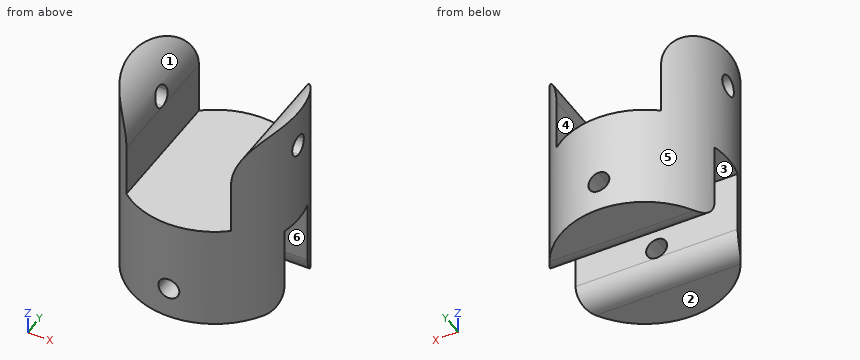
from build123d import *

# Parameters (mm, degrees)
F0_R        = 8
F1_DEPTH    = 10
F3_DEPTH    = 10
F5_DEPTH    = 8
F6_R        = 2
F7_T1_DEPTH = 37.4899959968
F9_DEPTH    = 12.5
F11_DEPTH   = 12.5


# Not quite as in the source:
# - a fillet or chamfer that OpenCascade refuses, or shapes differently, is made with other operations: its cross-section is extruded or revolved along the edge and cut away or added


with BuildPart() as f1:
    # F0 (on Top) → F1 (new body, symmetric)
    with BuildSketch(Plane.XY):
        Circle(F0_R)
    extrude(amount=F1_DEPTH, both=True)

    # F2 (on face) → F3 (cut)
    with BuildSketch(Plane.XY.offset(10)):
        with BuildLine():
            ThreePointArc((5, 6.2449979984), (0, 8), (-5, 6.2449979984))
            Line((-5, 6.2449979984), (-5, -6.2449979984))
            ThreePointArc((-5, -6.2449979984), (0, -8), (5, -6.2449979984))
            Line((5, -6.2449979984), (5, 6.2449979984))
        make_face()
    extrude(amount=-F3_DEPTH, mode=Mode.SUBTRACT)

    # F4 (on face) → F5 (cut)
    with BuildSketch(Plane(origin=(0, 0, -10), x_dir=(1, 0, 0), z_dir=(0, 0, -1))):
        with BuildLine():
            Line((7.7459666924, 2), (-7.7459666924, 2))
            ThreePointArc((-7.7459666924, 2), (-8, 0), (-7.7459666924, -2))
            Line((-7.7459666924, -2), (7.7459666924, -2))
            ThreePointArc((7.7459666924, -2), (7.9362375701, -1.0080343399), (8, 0))
            ThreePointArc((8, 0), (7.9362375701, 1.0080343399), (7.7459666924, 2))
        make_face()
    extrude(amount=-F5_DEPTH, mode=Mode.SUBTRACT)

    # F6
    f6_edges = [f1.edges().sort_by_distance(p)[0] for p in [
        (0, 2, -10),
        (0, -2, -10),
    ]]
    fillet(f6_edges, radius=F6_R)

    # F7: fillet of radius 5 on 2 edges, made by hand

    # F7_s2 → F7_t1 (cut)
    with BuildSketch(Plane.XZ.offset(-18.7449979984)):
        with BuildLine():
            ThreePointArc((-5, 5), (-6.4644660941, 8.5355339059), (-10, 10))
            Line((-10, 10), (-5, 10))
            Line((-5, 10), (-5, 5))
        make_face()
        with BuildLine():
            ThreePointArc((10, 10), (6.4644660941, 8.5355339059), (5, 5))
            Line((5, 5), (5, 10))
            Line((5, 10), (10, 10))
        make_face()
    extrude(amount=F7_T1_DEPTH, mode=Mode.SUBTRACT)

    # F8 (on Right) → F9 (cut, symmetric)
    with BuildSketch(Plane.YZ):
        with BuildLine():
            ThreePointArc((0, 5), (0.7071067812, 5.2928932188), (1, 6))
            ThreePointArc((1, 6), (-0.7071067812, 6.7071067812), (0, 5))
        make_face()
    extrude(amount=F9_DEPTH, both=True, mode=Mode.SUBTRACT)

    # F10 (on Front) → F11 (cut, symmetric)
    with BuildSketch(Plane.XZ):
        with BuildLine():
            ThreePointArc((0, -6), (-0.7071067812, -7.7071067812), (1, -7))
            ThreePointArc((1, -7), (0.7071067812, -6.2928932188), (0, -6))
        make_face()
    extrude(amount=F11_DEPTH, both=True, mode=Mode.SUBTRACT)


solid = f1.part
Check sheet for the modelled part. Datum: model origin and axes. Units: mm. Face numbers are marked on the shaded views. A direction names the side the tool comes from. Give positions to 0.01 mm unless a question says otherwise; leave off trailing zeros. Loops run counter-clockwise (first coordinate to the right, second up) from the corner with the lowest first, then second, coordinate; pieces in that order, holes last. Notation, with made-up numbers: M -17,-3 L 23,-3 A20 ccw 23,34 Z; hole C -13,-18.5 d11. An arc over 180 degrees is marked long. Answer as a JSON object with one key per item and string values. Group by question number.
Q1. Cross-section at C-C on x = -3.75. Record the cut outline in (y, z), then the cut area to 3 significant figures.
Q2. Cross-section at A-A on z = -2.25. Record the cut outline in (x, y), then the cut area to 3 significant figures.
Q3. Cross-section at B-B on y = 5.75. Record the cut outline in (x, z), then the cut area to 3 significant figures.
Q4. Cross-section at D-D on y = -1.5. Record the cut outline in (x, z), then the cut area to 3 significant figures.
Q5. Release check for a two-part mould opening along Y. For the marked faces 4, 5 and 6 record: released by +Y, released by -Y, zero draft, split by the parting line, or undercut.
Q6. Access from +Z, -Z, +X, -X, +Y, -Y to the whole of each face (thin tool, end or side, straight path). Record for the marked faces 1, 2 and 3.
Q7. Material ranges on line 1 along X through (y, z) = (-4, 3.25); line 2 along Z through (x, y) = (0, 6); line 3 along Z through (x, y) = (-6, 0), recorded low to high. Write a range as [from, to].
Q8. Go/stop test with flat-tipped pins: P1, Ø2.5, axis at y = 0, z = 6, coming from the -X side; P2, Ø2, axis at y = -4.5, z = 6, coming from the +X side; P3, Ø1, axis at x = -5, y = 2.5, coming from the -Z side; P4, Ø1, axis at x = -6, y = 3, coming from the +Z side. Record where each tip stops, or that it passes through.
Evaluation:
{
 "1": {"outline": "M -7.07,-10 L -4,-10 A2 ccw -2,-8 L -2,-2 L 2,-2 L 2,-8 A2 ccw 4,-10 L 7.07,-10 L 7.07,0 L -7.07,0 Z", "area": "108 mm2"},
 "2": {"outline": "M -7.75,-2 A8 ccw 7.75,-2 Z; M -7.75,2 L 7.75,2 A8 ccw Z", "area": "138 mm2"},
 "3": {"outline": "M -5.56,-10 L 5.56,-10 L 5.56,7.3 A5 ccw 5,5 L 5,0 L -5,0 L -5,5 A5 ccw -5.56,7.3 Z; hole C 0,-7 d2", "area": "115 mm2"},
 "4": {"outline": "M -7.86,-2 L 7.86,-2 L 7.86,9.52 A5 ccw 5,5 L 5,0 L -5,0 L -5,5 A5 ccw -7.86,9.52 Z", "area": "78.5 mm2"},
 "5": {"face 4": "zero draft", "face 5": "split by the parting line", "face 6": "undercut"},
 "6": {"face 1": "+Z, +Y, -Y", "face 2": "-Z, +X, -X, +Y, -Y", "face 3": "-Z, +X, -X"},
 "7": {"line 1": "x = [-6.93, -5], [5, 6.93]", "line 2": "z = [-10, -8], [-6, 0]", "line 3": "z = [-2, 5], [7, 8]"},
 "8": {"P1": "stops at x = -8", "P2": "stops at x = 7.19", "P3": "stops at z = -9.73", "P4": "stops at z = 8.57"}
}
